Work out the finished part from the listing and answer in its coordinate system (mm). Give positions to 0.01 mm unless a question says otherwise; leave off trailing zeros. Loops run counter-clockwise (first coordinate to the right, second up) from the corner with the lowest first, then second, coordinate; pieces in that order, holes last. Notation, with made-up numbers: (28, 71.5) - (39, 71.5) arc R26 cw to (39, 98.5) - close; hole circle Ø10 at (37, 45). An arc over 180 degrees is marked (long way). One line per question, with ' | ' between items. Start each with the question number.
1. Each of these flat-tipped pins is pushed along its axis until it touches: pin 1 (5 mm diameter, centred on y = -4, z = -60, fed in from -X); pin 2 (5 mm diameter, centred on y = -11.5, z = 13.5, fed in from +X); pin 3 (5 mm diameter, centred on y = -7, z = -48, fed in from -X). Where does it stop, or does it pass through?
2. Section D-D (z = -32) is taken. Determine the outline of the cut face in (x, y) (3 decimals), plus the area to 3 significant figures.
3. For a pull along X with two mould halves and no side action, classify faces 1 (the face through (-60.47, -6.574, -46.367)), 2 (the face through (-13.37, -6.57, 13.57)), 3 (the face through (-6, 0, -5)) as released by +X, released by -X, zero draft, split by the parting line, or undercut.
4. Section A-A (z = 0) is taken. Determine the outline of the cut face in (x, y) (3 decimals).
5. Find the intervals of material crossed by line 1 (Z direction, x = 0, y = -2.5); line 2 (Z direction, x = 53, y = -1.5); line 3 (X direction, y = -1.75, z = 2.5), in increasing order.
6. Section C-C (y = -7.25) is taken. Determine the outline of the cut face in (x, z), plus the area to 3 significant figures.
7. Section B-B (x = 61) is taken. Determine the outline of the cut face in (y, z) (3 decimals), plus the area to 3 significant figures.
from build123d import *

# Parameters (mm, degrees)
F0_R      = 76.2
F1_DEPTH  = 13.335
F3_DEPTH  = 13.336
F4_DEPTH  = 25.4
F5_R      = 19.05
F5_R_2    = 6.35
F6_DEPTH  = 13.335
F7_R      = 6.35
F8_DEPTH  = 25.4
F9_R      = 3.81
F10_DEPTH = 25.4


with BuildPart() as f1:
    # F0 (on Front) → F1 (new body)
    with BuildSketch(Plane.XZ):
        Circle(F0_R)
    extrude(amount=F1_DEPTH)

    # F2 (on face) → F3 (cut, through all)
    with BuildSketch(Plane.XZ.offset(13.335)):
        with BuildLine():
            Line((-5.08, 5.08), (-5.08, 69.598076))
            ThreePointArc((-5.08, 69.598076), (-48.103447, 48.081106), (-69.665028, 5.08))
            Line((-69.665028, 5.08), (-5.08, 5.08))
        make_face()
        with BuildLine():
            Line((5.08, 5.08), (69.665028, 5.08))
            ThreePointArc((69.665028, 5.08), (49.192924, 49.171714), (5.08, 69.598076))
            Line((5.08, 69.598076), (5.08, 5.08))
        make_face()
        with BuildLine():
            Line((8.76398, -5.08), (42.323278, -57.252949))
            ThreePointArc((42.323278, -57.252949), (60.579086, -33.766478), (68.451492, -5.08))
            Line((68.451492, -5.08), (8.76398, -5.08))
        make_face()
        with BuildLine():
            Line((0, -8.544917), (-33.414965, -61.338916))
            ThreePointArc((-33.414965, -61.338916), (0.192188, -68.934479), (33.709339, -60.951125))
            Line((33.709339, -60.951125), (0, -8.544917))
        make_face()
        with BuildLine():
            Line((-9.307793, -5.08), (-69.665028, -5.08))
            ThreePointArc((-69.665028, -5.08), (-61.51436, -33.874713), (-42.90387, -57.310125))
            Line((-42.90387, -57.310125), (-9.307793, -5.08))
        make_face()
    extrude(amount=-F3_DEPTH, mode=Mode.SUBTRACT)

    # F2 (on face) → F4 (cut)
    with BuildSketch(Plane.XZ.offset(13.335)):
        with BuildLine():
            Line((-5.08, 5.08), (-5.08, 69.598076))
            ThreePointArc((-5.08, 69.598076), (-48.103447, 48.081106), (-69.665028, 5.08))
            Line((-69.665028, 5.08), (-5.08, 5.08))
        make_face()
        with BuildLine():
            Line((5.08, 5.08), (69.665028, 5.08))
            ThreePointArc((69.665028, 5.08), (49.192924, 49.171714), (5.08, 69.598076))
            Line((5.08, 69.598076), (5.08, 5.08))
        make_face()
        with BuildLine():
            Line((8.76398, -5.08), (42.323278, -57.252949))
            ThreePointArc((42.323278, -57.252949), (60.579086, -33.766478), (68.451492, -5.08))
            Line((68.451492, -5.08), (8.76398, -5.08))
        make_face()
        with BuildLine():
            Line((0, -8.544917), (-33.414965, -61.338916))
            ThreePointArc((-33.414965, -61.338916), (0.192188, -68.934479), (33.709339, -60.951125))
            Line((33.709339, -60.951125), (0, -8.544917))
        make_face()
        with BuildLine():
            Line((-9.307793, -5.08), (-69.665028, -5.08))
            ThreePointArc((-69.665028, -5.08), (-61.51436, -33.874713), (-42.90387, -57.310125))
            Line((-42.90387, -57.310125), (-9.307793, -5.08))
        make_face()
    extrude(amount=-F4_DEPTH, mode=Mode.SUBTRACT)

    # F5 (on Front) → F6 (join)
    with BuildSketch(Plane.XZ):
        Circle(F5_R)
        Circle(F5_R_2, mode=Mode.SUBTRACT)
    extrude(amount=F6_DEPTH)

    # F7 (on face) → F8 (cut)
    with BuildSketch(Plane.XZ.offset(13.335)):
        Circle(F7_R)
    extrude(amount=-F8_DEPTH, mode=Mode.SUBTRACT)

    # F9 (on face) → F10 (cut)
    with BuildSketch(Plane.XZ.offset(13.335)):
        with Locations((48.26, 0)):
            Circle(F9_R)
    extrude(amount=-F10_DEPTH, mode=Mode.SUBTRACT)


solid = f1.part
Conclusion:
1) pin 1: x = -50 | pin 2: x = 75.4 | pin 3: x = -61.12
2) outline: (-69.155, -13.335) - (-62.443, -13.335) - (-62.443, 0) - (-69.155, 0) - close; (-26.624, -13.335) - (-14.845, -13.335) - (-14.845, 0) - (-26.624, 0) - close; (15.087, -13.335) - (26.08, -13.335) - (26.08, 0) - (15.087, 0) - close; (61.435, -13.335) - (69.155, -13.335) - (69.155, 0) - (61.435, 0) - close | area: 496 mm²
3) face 1: split by the parting line | face 2: undercut | face 3: zero draft
4) outline: (-76.2, -13.335) - (-6.35, -13.335) - (-6.35, 0) - (-76.2, 0) - close; (6.35, -13.335) - (44.45, -13.335) - (44.45, 0) - (6.35, 0) - close; (52.07, -13.335) - (76.2, -13.335) - (76.2, 0) - (52.07, 0) - close
5) line 1: -76.2 to -68.94, -19.05 to -6.35, 6.35 to 76.2 | line 2: -54.75 to -45.9, -5.08 to 5.08, 45.05 to 54.75 | line 3: -76.16 to -5.84, 5.84 to 45.38, 51.14 to 76.16
6) outline: circle Ø152.4 at (0, 0); hole (-69.67, -5.08) arc R76.2 ccw to (-42.9, -57.31) - (-14.2, -12.69) arc R19.05 cw to (-18.36, -5.08) - close; hole (-69.67, 5.08) - (-18.36, 5.08) arc R19.05 cw to (-5.08, 18.36) - (-5.08, 69.6) arc R76.2 ccw to start; hole (-33.41, -61.34) arc R76.2 ccw to (33.71, -60.95) - (6.11, -18.04) arc R19.05 cw to (-6.03, -18.07) - close; hole circle Ø12.7 at (0, 0); hole (5.08, 18.36) arc R19.05 cw to (18.36, 5.08) - (69.67, 5.08) arc R70.65 ccw to (5.08, 69.6) - close; hole (13.89, -13.04) - (42.32, -57.25) arc R76.2 ccw to (68.45, -5.08) - (18.36, -5.08) arc R19.05 cw to start; hole circle Ø7.62 at (48.26, 0) | area: 6,590 mm²
7) outline: (-13.335, -45.667) - (0, -45.667) - (0, -32.913) - (-13.335, -32.913) - close; (-13.335, -5.08) - (0, -5.08) - (0, 5.08) - (-13.335, 5.08) - close; (-13.335, 33.537) - (0, 33.537) - (0, 45.667) - (-13.335, 45.667) - close | area: 467 mm²
